from build123d import *

# Parameters (mm, degrees)
F0_W     = 63.523911
F0_H     = 39.456863
F1_DEPTH = 25
F2_R     = 7.543039
F3_DEPTH = 6.9
F4_W     = 13.097714
F4_H     = 13.097714
F5_DEPTH = 25


with BuildPart() as f1:
    # F0 (on Front) → F1 (new body)
    with BuildSketch(Plane.XZ):
        with Locations((31.761955, -19.728431)):
            Rectangle(F0_W, F0_H)
    extrude(amount=F1_DEPTH)

    # F2 (on face) → F3 (join)
    with BuildSketch(Plane.XY):
        with Locations((25.3403, -10.352623)):
            Circle(F2_R)
    extrude(amount=F3_DEPTH)

    # F4 (on face) → F5 (join)
    with BuildSketch(Plane.XY):
        with Locations((50.098749, -11.624221)):
            Rectangle(F4_W, F4_H)
    extrude(amount=F5_DEPTH)


solid = f1.part
Could you check a few things on this model? Use its own coordinates, in mm. A direction names the side the tool comes from. Give positions to 0.01 mm unless a question says otherwise; leave off trailing zeros. Order: outer loops, then holes, each group sorted by start corner. A loop starts at its lowest first (then second) coordinate and runs counter-clockwise, first axis right, second up.
1. Suppose I cut it at D-D (x = 31). List the corners of the cut face in (y, z) for me.
2. We'd pull the mould along X, two halves only. Please class faces 5 (the flat face through (0, -12, -20)), 6 (the flat face through (43.55, -12, 12)), 7 (the flat face through (50, -12, 25)): pulls with the +X half, pulls with the -X half, needs draft (parallel to the pull), parting line crosses it, or undercut.
3. Suppose I cut it at A-A (x = 48). List the corners of the cut face in (y, z) for me.
4. Suppose I cut it at C-C (y = -8.75). List the corners of the cut face in (x, z) for me.
5. Suppose I cut it at B-B (z = 2.5). List the corners of the cut face in (x, y) for me, plus the area to 3 significant figures.
6. I need wall thicknesses on L1, parallel to Z at x = 55, y = -19.75; L2, parallel to X at y = -11.5, z = 22.5; L3, parallel to Z at x = 20.5, y = -12. Which ranges of each line are inside material? Lowest first, please.
7. Will these pins go through, and if not, where does the flat tip stop? P1, Ø6.5, axis at y = -10.5, z = 14, coming from the +X side; P2, Ø4.5, axis at x = 22.5, y = -9, coming from the +Z side; P3, Ø5, axis at x = 40.5, y = -13.5, coming from the +Z side; P4, Ø5, axis at x = 26.5, z = 10.5, coming from the +Y side (1 decimal).
8. For faces 1 (the cylindrical face through (19.781, -5.255, 3.402)), 2 (the flat face through (56.648, -12, 12)), 3 (the flat face through (25, -10, 6.9)), 4 (the flat face through (50, -5.075, 12)), which set-ups out of +Z, -Z, +X, -X, +Y, -Y let a thin tool reach every point of the face, with its end or its side?
Solved:
1. outline: (-25, -39.46) - (0, -39.46) - (0, 0) - (-5.37, 0) - (-5.37, 6.9) - (-15.34, 6.9) - (-15.34, 0) - (-25, 0) - close
2. face 5: pulls with the -X half
2. face 6: undercut
2. face 7: needs draft
3. outline: (-25, -39.46) - (0, -39.46) - (0, 0) - (-5.08, 0) - (-5.08, 25) - (-18.17, 25) - (-18.17, 0) - (-25, 0) - close
4. outline: (0, -39.46) - (63.52, -39.46) - (63.52, 0) - (56.65, 0) - (56.65, 25) - (43.55, 25) - (43.55, 0) - (32.71, 0) - (32.71, 6.9) - (17.97, 6.9) - (17.97, 0) - (0, 0) - close
5. outline: circle Ø15.09 at (25.34, -10.35); (43.55, -18.17) - (56.65, -18.17) - (56.65, -5.08) - (43.55, -5.08) - close
5. area: 350 mm2
6. L1: z = -39.46 to 0
6. L2: x = 43.55 to 56.65
6. L3: z = -39.46 to 6.9
7. P1: stops at x = 56.65
7. P2: stops at z = 6.9
7. P3: stops at z = 0
7. P4: passes through
8. face 1: +Z
8. face 2: +Z, +X, +Y, -Y
8. face 3: +Z, -X, +Y, -Y
8. face 4: +Z, +X, +Y
